The model under review builds one solid part; all positions refer to its coordinate system, in mm. Face numbers are marked on the shaded views. A direction names the side the tool comes from. Give positions to 0.01 mm unless a question says otherwise; leave off trailing zeros. Write each loop counter-clockwise with the first axis right and the second up, starting at its lowest first coordinate (ties: lowest second). Pieces come first, ordered by that corner, then holes.
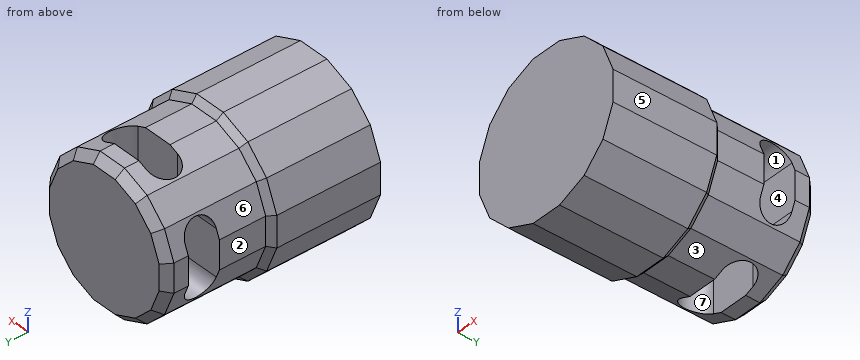
from build123d import *

# Parameters (mm, degrees)
BOSS_EXTRUDE1_DEPTH            = 50
BOSS_EXTRUDE2_DEPTH            = 55
CHAMFER1_SIZE                  = 4
CHAMFER3_SIZE                  = 3
CUT_EXTRUDE1_REACH             = 79.891
CUT_EXTRUDE1_DIRECTION_2_REACH = 79.891
CUT_EXTRUDE2_REACH             = 79.891
CUT_EXTRUDE2_DIRECTION_2_REACH = 79.891


with BuildPart() as part:
    # Sketch1 → Boss-Extrude1 (new body)
    with BuildSketch(Plane(origin=(0, 0, 0), x_dir=(1, 0, 0), z_dir=(0, 1, 0))):
        Polygon((36, 7.160845226), (30.519326341, 20.392361905), (20.392361905, 30.519326341), (7.160845226, 36), (-7.160845226, 36), (-20.392361905, 30.519326341), (-30.519326341, 20.392361905), (-36, 7.160845226), (-36, -7.160845226), (-30.519326341, -20.392361905), (-20.392361905, -30.519326341), (-7.160845226, -36), (7.160845226, -36), (20.392361905, -30.519326341), (30.519326341, -20.392361905), (36, -7.160845226), align=None)
    extrude(amount=BOSS_EXTRUDE1_DEPTH)

    # Sketch2 → Boss-Extrude2 (add)
    with BuildSketch(Plane.XZ):
        Polygon((33.062603536, 22.091725397), (22.091725397, 33.062603536), (7.757582328, 39), (-7.757582328, 39), (-22.091725397, 33.062603536), (-33.062603536, 22.091725397), (-39, 7.757582328), (-39, -7.757582328), (-33.062603536, -22.091725397), (-22.091725397, -33.062603536), (-7.757582328, -39), (7.757582328, -39), (22.091725397, -33.062603536), (33.062603536, -22.091725397), (39, -7.757582328), (39, 7.757582328), align=None)
    extrude(amount=BOSS_EXTRUDE2_DEPTH)

    # Chamfer1
    chamfer1_edges = [part.edges().sort_by_distance(p)[0] for p in [
        (25.455844123, 50, -25.455844123),
        (13.776603565, 50, -33.25966317),
        (0, 50, -36),
        (-13.776603565, 50, -33.25966317),
        (-25.455844123, 50, -25.455844123),
        (-33.25966317, 50, -13.776603565),
        (-36, 50, 0),
        (-33.25966317, 50, 13.776603565),
        (-25.455844123, 50, 25.455844123),
        (-13.776603565, 50, 33.25966317),
        (36, 50, 0),
        (0, 50, 36),
        (13.776603565, 50, 33.25966317),
        (25.455844123, 50, 25.455844123),
        (33.25966317, 50, 13.776603565),
        (33.25966317, 50, -13.776603565),
    ]]
    chamfer(chamfer1_edges, length=CHAMFER1_SIZE)

    # Chamfer3
    chamfer3_edges = [part.edges().sort_by_distance(p)[0] for p in [
        (36.031301768, 0, 14.924653862),
        (27.577164466, 0, 27.577164466),
        (14.924653862, 0, 36.031301768),
        (0, 0, 39),
        (-14.924653862, 0, 36.031301768),
        (-27.577164466, 0, 27.577164466),
        (-36.031301768, 0, 14.924653862),
        (-39, 0, 0),
        (-36.031301768, 0, -14.924653862),
        (-27.577164466, 0, -27.577164466),
        (-14.924653862, 0, -36.031301768),
        (0, 0, -39),
        (14.924653862, 0, -36.031301768),
        (27.577164466, 0, -27.577164466),
        (36.031301768, 0, -14.924653862),
        (39, 0, 0),
    ]]
    chamfer(chamfer3_edges, length=CHAMFER3_SIZE - 0.0001)  # a hair under: the kernel refuses the full size

    # Cut-Extrude1: up to this face of the body (flat: up to its plane)
    cut_extrude1_end = Plane(part.part.faces().sort_by_distance((0, 23, -36))[0])
    # Sketch3 → Cut-Extrude1 (cut, up to the picked face)
    with BuildSketch(Plane.XY, mode=Mode.PRIVATE) as cut_extrude1_sk1:
        with BuildLine():
            Line((-11.5, 38.8), (11.5, 38.8))
            ThreePointArc((11.5, 38.8), (19.3, 31), (11.5, 23.2))
            Line((11.5, 23.2), (-11.5, 23.2))
            ThreePointArc((-11.5, 23.2), (-19.3, 31), (-11.5, 38.8))
        make_face()
    cut_extrude1_tool1 = split(extrude(cut_extrude1_sk1.sketch, amount=-CUT_EXTRUDE1_REACH, mode=Mode.PRIVATE), bisect_by=cut_extrude1_end, keep=Keep.BOTH, mode=Mode.PRIVATE)
    add(cut_extrude1_tool1.solids().sort_by(Axis((0, 31, 0), (0, 0, -1)))[0], mode=Mode.SUBTRACT)

    # Cut-Extrude1 direction 2: up to this face of the body (flat: up to its plane)
    cut_extrude1_direction_2_end = Plane(part.part.faces().sort_by_distance((0, 23, 36))[0])
    # Sketch3 → Cut-Extrude1 direction 2 (cut, up to the picked face)
    with BuildSketch(Plane.XY, mode=Mode.PRIVATE) as cut_extrude1_direction_2_sk1:
        with BuildLine():
            Line((-11.5, 38.8), (11.5, 38.8))
            ThreePointArc((11.5, 38.8), (19.3, 31), (11.5, 23.2))
            Line((11.5, 23.2), (-11.5, 23.2))
            ThreePointArc((-11.5, 23.2), (-19.3, 31), (-11.5, 38.8))
        make_face()
    cut_extrude1_direction_2_tool1 = split(extrude(cut_extrude1_direction_2_sk1.sketch, amount=CUT_EXTRUDE1_DIRECTION_2_REACH, mode=Mode.PRIVATE), bisect_by=cut_extrude1_direction_2_end, keep=Keep.BOTH, mode=Mode.PRIVATE)
    add(cut_extrude1_direction_2_tool1.solids().sort_by(Axis((0, 31, 0), (0, 0, 1)))[0], mode=Mode.SUBTRACT)

    # Cut-Extrude2: up to this face of the body (flat: up to its plane)
    cut_extrude2_end = Plane(part.part.faces().sort_by_distance((36, 23, 0))[0])
    # Sketch4 → Cut-Extrude2 (cut, up to the picked face)
    with BuildSketch(Plane(origin=(0, 0, 0), x_dir=(0, 0, -1), z_dir=(1, 0, 0)), mode=Mode.PRIVATE) as cut_extrude2_sk1:
        with BuildLine():
            Line((-11.5, 38.8), (11.5, 38.8))
            ThreePointArc((11.5, 38.8), (19.3, 31), (11.5, 23.2))
            Line((11.5, 23.2), (-11.5, 23.2))
            ThreePointArc((-11.5, 23.2), (-19.3, 31), (-11.5, 38.8))
        make_face()
    cut_extrude2_tool1 = split(extrude(cut_extrude2_sk1.sketch, amount=CUT_EXTRUDE2_REACH, mode=Mode.PRIVATE), bisect_by=cut_extrude2_end, keep=Keep.BOTH, mode=Mode.PRIVATE)
    add(cut_extrude2_tool1.solids().sort_by(Axis((0, 31, 0), (1, 0, 0)))[0], mode=Mode.SUBTRACT)

    # Cut-Extrude2 direction 2: up to this face of the body (flat: up to its plane)
    cut_extrude2_direction_2_end = Plane(part.part.faces().sort_by_distance((-36, 23, 0))[0])
    # Sketch4 → Cut-Extrude2 direction 2 (cut, up to the picked face)
    with BuildSketch(Plane(origin=(0, 0, 0), x_dir=(0, 0, -1), z_dir=(1, 0, 0)), mode=Mode.PRIVATE) as cut_extrude2_direction_2_sk1:
        with BuildLine():
            Line((-11.5, 38.8), (11.5, 38.8))
            ThreePointArc((11.5, 38.8), (19.3, 31), (11.5, 23.2))
            Line((11.5, 23.2), (-11.5, 23.2))
            ThreePointArc((-11.5, 23.2), (-19.3, 31), (-11.5, 38.8))
        make_face()
    cut_extrude2_direction_2_tool1 = split(extrude(cut_extrude2_direction_2_sk1.sketch, amount=-CUT_EXTRUDE2_DIRECTION_2_REACH, mode=Mode.PRIVATE), bisect_by=cut_extrude2_direction_2_end, keep=Keep.BOTH, mode=Mode.PRIVATE)
    add(cut_extrude2_direction_2_tool1.solids().sort_by(Axis((0, 31, 0), (-1, 0, 0)))[0], mode=Mode.SUBTRACT)


solid = part.part
1) To check wall thickness, follow probe 1 along Y at (x, z) = (-12, -25); probe 2 along X at (y, z) = (37, 25); probe 3 along Y at (x, z) = (29, -16.5). State the ranges of each line that lie inside material, in increasing order.
2) The part is to be moulded in two halves that separate along X. For the marked faces 5, 6 and 7, say which applies: +X half, -X half, draft (parallel to the pull), parting line (faces both ways), or undercut.
3) Tool access review of the marked faces 1, 2, 3 and 4: name each direction out of +Z, -Z, +X, -X, +Y, -Y from which nothing blocks a thin tool from reaching the whole face with its end or side.
4) Consider section D-D, the plane y = 31. Give the boundary of the cut face in (x, z), then the cut area to 3 significant figures.
5) Consider section C-C, the plane y = -46. Give the boundary of the cut face in (x, z).
6) Insertion check: pin 1 (7 mm diameter, centred on y = 6, z = 0.5, fed in from +X); pin 2 (5 mm diameter, centred on y = -13, z = 12.5, fed in from +X); pin 3 (1 mm diameter, centred on y = -9.5, z = -17, fed in from +X). Each pin has a flat end and moves straight along its axis. Give the tip position at first contact, or say it passes through.
Answer block:
1. probe 1: y = -55 to 23.22, 38.78 to 50
1. probe 2: x = -25.91 to -16.48, 16.48 to 25.91
1. probe 3: y = -55 to 25.01, 36.99 to 48.89
2. face 5: +X half
2. face 6: -X half
2. face 7: undercut
3. face 1: +X, -X
3. face 2: +Z, -Z, -X, +Y
3. face 3: -Z, +X, +Y
3. face 4: none
4. outline: (-30.97, -19.3) - (-30.52, -20.39) - (-20.39, -30.52) - (-19.3, -30.97) - (-19.3, -19.3) - close; (-30.97, 19.3) - (-19.3, 19.3) - (-19.3, 30.97) - (-20.39, 30.52) - (-30.52, 20.39) - close; (19.3, -30.97) - (20.39, -30.52) - (30.52, -20.39) - (30.97, -19.3) - (19.3, -19.3) - close; (19.3, 19.3) - (30.97, 19.3) - (30.52, 20.39) - (20.39, 30.52) - (19.3, 30.97) - close
4. area: 300 mm2
5. outline: (-39, -7.76) - (-33.06, -22.09) - (-22.09, -33.06) - (-7.76, -39) - (7.76, -39) - (22.09, -33.06) - (33.06, -22.09) - (39, -7.76) - (39, 7.76) - (33.06, 22.09) - (22.09, 33.06) - (7.76, 39) - (-7.76, 39) - (-22.09, 33.06) - (-33.06, 22.09) - (-39, 7.76) - close
6. pin 1: stops at x = 36
6. pin 2: stops at x = 38.07
6. pin 3: stops at x = 35.38
